The listing builds one solid part. Answer for the finished solid, in the listing's coordinates (mm). A direction names the side the tool comes from. Give positions to 0.01 mm unless a question says otherwise; leave off trailing zeros. Write each question's results on one line, items separated by ' | '. Start each with the question number.
Q1. Find the intervals of material crossed by probe 1 along Z at (x, y) = (4, -10.75) (3 decimals); probe 2 along X at (y, z) = (4.75, -20); probe 3 along X at (y, z) = (2.7, 9), in increasing order.
Q2. For a pull along Z with two mould halves and no side action, classify faces 5 (the face through (-3.442, 6.607, 18.918)), 6 (the face through (-3.55, 6.61, 31.02)), 7 (the face through (0, -12.5, -13)) as pulls with the +Z half, pulls with the -Z half, needs draft (parallel to the pull), parting line crosses it, or undercut.
Q3. Flat-ended cylindrical pins translate along their axes: pin 1 Ø2 at (x, y) = (36, 6.5) entering from -Z; pin 2 Ø3 at (x, z) = (-27.5, -13) entering from -Y; pin 3 Ø2.5 at (x, y) = (-4, -10) entering from -Z. Find the tip coordinate at first contact, or state that the pin passes through.
Q4. For faces 1 (the face through (-0.1, -5.325, -29.3)), 2 (the face through (6.495, 3, -25)), 3 (the face through (10, -3, 25)), 4 (the face through (10, -3, -25)), determine the directions among +Z, -Z, +X, -X, +Y, -Y from which every point of the face is accessible in a straight line to the end or side of a thin tool.
Q5. Section A-A (x = 20) is taken. State how many separate pieces and enclosed holes the cut face has, plus the area to 3 significant figures.
```python
from build123d import *

# Parameters (mm, degrees)
SKETCH_1_R          = 55
EXTRUDE_1_DEPTH     = 5
SKETCH_2_R          = 52.4
EXTRUDE_2_DEPTH     = 3
SKETCH_3_W          = 35
SKETCH_3_H          = 30
EXTRUDE_3_DEPTH     = 25
SKETCH_5_R          = 4.1
CUT_EXTRUDE_2_DEPTH = 9
SKETCH_6_R          = 2.75
CUT_EXTRUDE_3_DEPTH = 34
SKETCH2_W           = 20.25
SKETCH2_H           = 10.35
CUT_EXTRUDE1_DEPTH  = 73.5
SKETCH3_W           = 17.5
SKETCH3_H           = 27.9
SKETCH3_W_2         = 48.4
SKETCH3_H_2         = 25.4
CUT_EXTRUDE2_DEPTH  = 4
CHAMFER1_SIZE       = 2
CHAMFER1_SIZE2      = 0.535898385
SKETCH4_W           = 35
SKETCH4_H           = 30
CUT_EXTRUDE3_DEPTH  = 12.5
BOSS_EXTRUDE2_START = -2
SKETCH5_W           = 20
SKETCH5_H           = 70
BOSS_EXTRUDE2_DEPTH = 5.325
SKETCH6_R           = 4.15
CUT_EXTRUDE4_DEPTH  = 14.325
CUT_EXTRUDE5_DEPTH  = 6.5
CHAMFER2_SIZE       = 1
CHAMFER2_SIZE2      = 2.747477419
SKETCH8_R           = 1.5
CUT_EXTRUDE6_DEPTH  = 17.5
CHAMFER3_SIZE       = 1
CHAMFER3_SIZE2      = 1.732050808


with BuildPart() as part:
    # Эскиз1 → Бобышка-Вытянуть1 (new body)
    with BuildSketch(Plane(origin=(0, 0, 0), x_dir=(1, 0, 0), z_dir=(0, 1, 0))):
        with Locations(Location((0, 0, 0), (0, 0, 270))):  # turned: the seam where the file's is
            Circle(SKETCH_1_R)
    extrude(amount=EXTRUDE_1_DEPTH)

    # Эскиз2 → Бобышка-Вытянуть2 (add)
    with BuildSketch(Plane(origin=(0, 5, 0), x_dir=(1, 0, 0), z_dir=(0, 1, 0))):
        with Locations(Location((0, 0, 0), (0, 0, 270))):  # turned: the seam where the file's is
            Circle(SKETCH_2_R)
    extrude(amount=EXTRUDE_2_DEPTH)

    # Эскиз3 → Бобышка-Вытянуть3 (add)
    with BuildSketch(Plane.XZ):
        Rectangle(SKETCH_3_W, SKETCH_3_H)
    extrude(amount=EXTRUDE_3_DEPTH)

    # Эскиз5 → Вырез-Вытянуть2 (cut, through all)
    with BuildSketch(Plane.XZ):
        with Locations(Location((33.234018716, -33.234018716, 0), (0, 0, 270))):  # turned: the seam where the file's is
            Circle(SKETCH_5_R)
        with Locations(Location((-33.234018716, -33.234018716, 0), (0, 0, 270))):  # turned: the seam where the file's is
            Circle(SKETCH_5_R)
        with Locations(Location((-33.234018716, 33.234018716, 0), (0, 0, 270))):  # turned: the seam where the file's is
            Circle(SKETCH_5_R)
        with Locations(Location((33.234018716, 33.234018716, 0), (0, 0, 270))):  # turned: the seam where the file's is
            Circle(SKETCH_5_R)
    extrude(amount=-CUT_EXTRUDE_2_DEPTH, mode=Mode.SUBTRACT)

    # Эскиз6 → Вырез-Вытянуть3 (cut, through all)
    with BuildSketch(Plane(origin=(0, 8, 0), x_dir=(1, 0, 0), z_dir=(0, 1, 0))):
        with Locations(Location((-18, 20, 0), (0, 0, 270))):  # turned: the seam where the file's is
            Circle(SKETCH_6_R)
    extrude(amount=-CUT_EXTRUDE_3_DEPTH, mode=Mode.SUBTRACT)

    # Sketch2 → Cut-Extrude1 (cut, through all)
    with BuildSketch(Plane.ZY.offset(17.5)):
        with Locations((0, -12.5)):
            Rectangle(SKETCH2_W, SKETCH2_H)
    extrude(amount=-CUT_EXTRUDE1_DEPTH, mode=Mode.SUBTRACT)

    # Sketch3 → Cut-Extrude2 (cut)
    with BuildSketch(Plane(origin=(0, 8, 0), x_dir=(1, 0, 0), z_dir=(0, 1, 0))):
        with Locations((35, 0)):
            Rectangle(SKETCH3_W, SKETCH3_H)
        Rectangle(SKETCH3_W_2, SKETCH3_H_2)
    extrude(amount=-CUT_EXTRUDE2_DEPTH, mode=Mode.SUBTRACT)

    # Chamfer1
    chamfer1_edges = [part.edges().sort_by_distance(p)[0] for p in [
        (0, 8, -52.4),
    ]]
    chamfer1_side = [part.faces().sort_by_distance(p)[0] for p in [
        (0, 6.5, -52.4),
    ]]
    chamfer(chamfer1_edges, length=CHAMFER1_SIZE, length2=CHAMFER1_SIZE2, reference=chamfer1_side[0])

    # Sketch4 → Cut-Extrude3 (cut)
    with BuildSketch(Plane.XZ.offset(25)):
        Rectangle(SKETCH4_W, SKETCH4_H)
    extrude(amount=-CUT_EXTRUDE3_DEPTH, mode=Mode.SUBTRACT)

    # Sketch5 → Boss-Extrude2 (add)
    with BuildSketch(Plane.XZ.offset(7.325).offset(BOSS_EXTRUDE2_START)):
        Rectangle(SKETCH5_W, SKETCH5_H)
    extrude(amount=-BOSS_EXTRUDE2_DEPTH)

    # Sketch6 → Cut-Extrude4 (cut, through all)
    with BuildSketch(Plane.XZ.offset(5.325)):
        with Locations(Location((0, 25, 0), (0, 0, 270))):  # turned: the seam where the file's is
            Circle(SKETCH6_R)
        with Locations(Location((0, -25, 0), (0, 0, 270))):  # turned: the seam where the file's is
            Circle(SKETCH6_R)
    extrude(amount=-CUT_EXTRUDE4_DEPTH, mode=Mode.SUBTRACT)

    # Sketch7 → Cut-Extrude5 (cut)
    with BuildSketch(Plane(origin=(0, 8, 0), x_dir=(1, 0, 0), z_dir=(0, 1, 0))):
        Polygon((0, -32.5), (6.495190528, -28.75), (6.495190528, -21.25), (0, -17.5), (-6.495190528, -21.25), (-6.495190528, -28.75), align=None)
        Polygon((0, 17.5), (6.495190528, 21.25), (6.495190528, 28.75), (0, 32.5), (-6.495190528, 28.75), (-6.495190528, 21.25), align=None)
    extrude(amount=-CUT_EXTRUDE5_DEPTH, mode=Mode.SUBTRACT)

    # Chamfer2
    chamfer2_edges = [part.edges().sort_by_distance(p)[0] for p in [
        (-3.247595264, 8, 30.625),
        (3.247595264, 8, 30.625),
        (6.495190528, 8, 25),
        (3.247595264, 8, 19.375),
        (-3.247595264, 8, 19.375),
        (-6.495190528, 8, 25),
        (-3.247595264, 8, -19.375),
        (3.247595264, 8, -19.375),
        (6.495190528, 8, -25),
        (3.247595264, 8, -30.625),
        (-3.247595264, 8, -30.625),
        (-6.495190528, 8, -25),
    ]]
    chamfer2_side = [part.faces().sort_by_distance(p)[0] for p in [
        (0, 8, -50.397163297),
    ]]
    chamfer(chamfer2_edges, length=CHAMFER2_SIZE, length2=CHAMFER2_SIZE2, reference=chamfer2_side[0])

    # Sketch8 → Cut-Extrude6 (cut, through all)
    with BuildSketch(Plane(origin=(0, 4, 0), x_dir=(1, 0, 0), z_dir=(0, 1, 0))):
        with Locations(Location((20, 9, 0), (0, 0, 270))):  # turned: the seam where the file's is
            Circle(SKETCH8_R)
        with Locations(Location((20, -9, 0), (0, 0, 270))):  # turned: the seam where the file's is
            Circle(SKETCH8_R)
        with Locations(Location((-20, 9, 0), (0, 0, 270))):  # turned: the seam where the file's is
            Circle(SKETCH8_R)
        with Locations(Location((-20, -9, 0), (0, 0, 270))):  # turned: the seam where the file's is
            Circle(SKETCH8_R)
    extrude(amount=-CUT_EXTRUDE6_DEPTH, mode=Mode.SUBTRACT)

    # Chamfer3
    chamfer3_edges = [part.edges().sort_by_distance(p)[0] for p in [
        (24.2, 8, 0),
        (0, 8, -12.7),
        (-24.2, 8, 0),
        (0, 8, 12.7),
    ]]
    chamfer3_side = [part.faces().sort_by_distance(p)[0] for p in [
        (-4.481064423, 8, 32.761431253),
    ]]
    chamfer(chamfer3_edges, length=CHAMFER3_SIZE, length2=CHAMFER3_SIZE2, reference=chamfer3_side[0])


solid = part.part
```
Answers below:
1) probe 1: z = -15 to -10.125, 10.125 to 15 | probe 2: x = -51.23 to -20.75, -15.25 to -4.33, 4.33 to 51.23 | probe 3: x = -54.26 to -21.5, -18.5 to 18.5, 21.5 to 54.26
2) face 5: undercut | face 6: undercut | face 7: needs draft
3) pin 1: stops at z = -38.89 | pin 2: stops at y = 0 | pin 3: stops at z = -15
4) face 1: -Z, +X, -X, -Y | face 2: +Y | face 3: +Z, +X, -Y | face 4: -Z, +X, -Y
5) separate pieces: 3 | enclosed holes: 0 | area: 674 mm2
